Can you work these out from the drawing? Everything is in mm from the part's minimum corner. Round coordinates to 2 decimals unless told otherwise and drop trailing zeros. Write each loop counter-clockwise with the first axis right and the second up, starting at its lowest first coordinate (ties: lowest second). Pieces come first, ordered by that corner, then holes. Notation, with made-up numbers: M 37.25,19 L 55.25,19 A16 ccw 55.25,27 Z; hole C 44.5,27.5 d10. An arc over 180 degrees is marked long. Answer in a Markdown table with one row per item. Add a question column.
(1) If I drill on probe 1 along X at (y, z) = (8.5, 0.7); probe 2 along X at (y, z) = (4.75, 0.5), over which ranges is the centre line in solid material (lowest first)?
(2) I'm going to push a flat-ended pin straight in: pin 1 (1 mm diameter, centred on x = 4.5, y = 4.5, fed in from -Z). Where does the tip first touch, or does it pass through?
(3) If we mould it in two halves opening along X, with no side actions, what happens to the marked faces 1, 2 and 3? For each: released by +X, released by -X, zero draft, split by the parting line, or undercut.
(4) Suppose I cut it at C-C, the plane z = 1. Write out the boundary of the cut face in (x, y), then the cut area to 3 significant figures.
(5) Suppose I cut it at A-A, the plane x = 8.5. Write out the boundary of the cut face in (y, z), then the cut area to 3 significant figures.
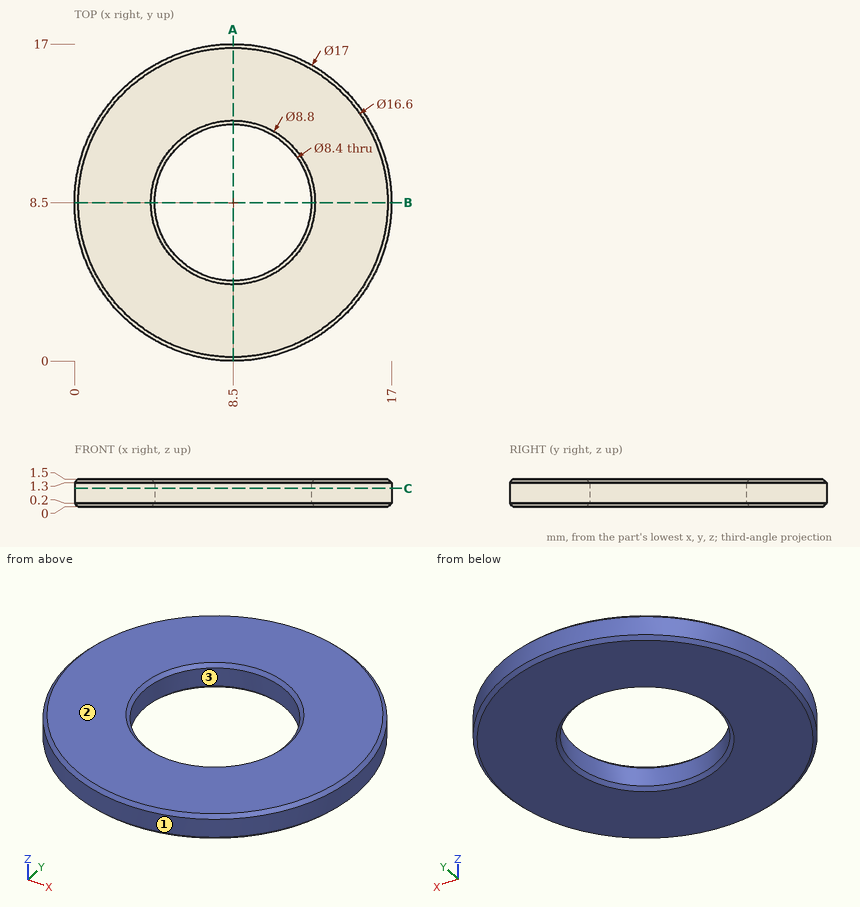
Calculated:
| question | item | result |
|---|---|---|
| 1 | probe 1 | 0 to 4.3, 12.7 to 17 |
| 1 | probe 2 | 0.87 to 6.61, 10.39 to 16.13 |
| 2 | pin 1 | z = 0 |
| 3 | face 1 | split by the parting line |
| 3 | face 2 | zero draft |
| 3 | face 3 | undercut |
| 4 | outline | C 8.5,8.5 d17; hole C 8.5,8.5 d8.4 |
| 4 | area | 172 mm² |
| 5 | outline | M 0,0.2 L 0.2,0 L 4.1,0 L 4.3,0.2 L 4.3,1.3 L 4.1,1.5 L 0.2,1.5 L 0,1.3 Z; M 12.7,0.2 L 12.9,0 L 16.8,0 L 17,0.2 L 17,1.3 L 16.8,1.5 L 12.9,1.5 L 12.7,1.3 Z |
| 5 | area | 12.7 mm² |
